from build123d import *

# Parameters (mm, degrees)
SKETCH_1_R             = 60
SM_BASE_FLANGE_1_DEPTH = 2
CUT_EXTRUDE_1_REACH    = 86.876
SKETCH_6_R             = 1.5


# Sheet-metal steps are written as plain solids
with BuildPart() as part:
    # Sketch 1 → 基体-法兰1 (new body)
    with BuildSketch(Plane(origin=(0, 0, 0), x_dir=(1, 0, 0), z_dir=(0, 1, 0))):
        with Locations(Location((0, 0, 0), (0, 0, 270))):
            Circle(SKETCH_1_R)
        with BuildLine():
            Line((-5.662691153, -45.650125179), (-5.41648719, -43.665337128))
            ThreePointArc((-5.41648719, -43.665337128), (-0.000329002, 43.999999999), (5.41714019, -43.665256122))
            Line((5.41714019, -43.665256122), (5.663373835, -45.650040491))
            ThreePointArc((5.663373835, -45.650040491), (0.000343957, -45.999999999), (-5.662691153, -45.650125179))
        make_face(mode=Mode.SUBTRACT)
    extrude(amount=-SM_BASE_FLANGE_1_DEPTH)

    # 草图6 → 切除-拉伸1 (cut, up to next)
    with BuildSketch(Plane(origin=(0, 0, 0), x_dir=(1, 0, 0), z_dir=(0, 1, 0)), mode=Mode.PRIVATE) as cut_extrude_1_sk1:
        with Locations(Location((36.769552622, 36.769552622, 0), (0, 0, 270))):
            Circle(SKETCH_6_R)
    cut_extrude_1_tool1 = extrude(cut_extrude_1_sk1.sketch, amount=-CUT_EXTRUDE_1_REACH, mode=Mode.PRIVATE) & part.part
    # 草图6 → 切除-拉伸1 (cut, up to next)
    with BuildSketch(Plane(origin=(0, 0, 0), x_dir=(1, 0, 0), z_dir=(0, 1, 0)), mode=Mode.PRIVATE) as cut_extrude_1_sk2:
        with Locations(Location((-36.769552622, 36.769552622, 0), (0, 0, 270))):
            Circle(SKETCH_6_R)
    cut_extrude_1_tool2 = extrude(cut_extrude_1_sk2.sketch, amount=-CUT_EXTRUDE_1_REACH, mode=Mode.PRIVATE) & part.part
    # 草图6 → 切除-拉伸1 (cut, up to next)
    with BuildSketch(Plane(origin=(0, 0, 0), x_dir=(1, 0, 0), z_dir=(0, 1, 0)), mode=Mode.PRIVATE) as cut_extrude_1_sk3:
        with Locations(Location((36.769552622, -36.769552622, 0), (0, 0, 270))):
            Circle(SKETCH_6_R)
    cut_extrude_1_tool3 = extrude(cut_extrude_1_sk3.sketch, amount=-CUT_EXTRUDE_1_REACH, mode=Mode.PRIVATE) & part.part
    # 草图6 → 切除-拉伸1 (cut, up to next)
    with BuildSketch(Plane(origin=(0, 0, 0), x_dir=(1, 0, 0), z_dir=(0, 1, 0)), mode=Mode.PRIVATE) as cut_extrude_1_sk4:
        with Locations(Location((-36.769552622, -36.769552622, 0), (0, 0, 270))):
            Circle(SKETCH_6_R)
    cut_extrude_1_tool4 = extrude(cut_extrude_1_sk4.sketch, amount=-CUT_EXTRUDE_1_REACH, mode=Mode.PRIVATE) & part.part
    add(cut_extrude_1_tool1.solids().sort_by_distance((36.769553, 0, -36.769553))[0], mode=Mode.SUBTRACT)
    add(cut_extrude_1_tool2.solids().sort_by_distance((-36.769553, 0, -36.769553))[0], mode=Mode.SUBTRACT)
    add(cut_extrude_1_tool3.solids().sort_by_distance((36.769553, 0, 36.769553))[0], mode=Mode.SUBTRACT)
    add(cut_extrude_1_tool4.solids().sort_by_distance((-36.769553, 0, 36.769553))[0], mode=Mode.SUBTRACT)


solid = part.part
Model file for the job. Use its own axes, mm. Round coordinates to 2 decimals unless told otherwise and drop trailing zeros. Loops run counter-clockwise (first coordinate to the right, second up) from the corner with the lowest first, then second, coordinate; pieces in that order, holes last.
1. Band-saw the part on A-A, the plane x = 0. List the corners of the cut face in (y, z), and give its area (3 significant figures).
Check values:
outline: (-2, -60) - (0, -60) - (0, -44) - (-2, -44) - close; (-2, 46) - (0, 46) - (0, 60) - (-2, 60) - close
area: 60.0 mm2
2. Band-saw the part on C-C, the plane y = -1.5. List the corners of the cut face in (x, z).
Check values:
outline: circle Ø120 at (0, 0); hole circle Ø3 at (-36.77, -36.77); hole circle Ø3 at (-36.77, 36.77); hole (-5.66, 45.65) - (-5.42, 43.67) arc R44 ccw (long way) to (5.42, 43.67) - (5.66, 45.65) arc R46 ccw to start; hole circle Ø3 at (36.77, -36.77); hole circle Ø3 at (36.77, 36.77)
3. Wall check: probe 1 along X at (y, z) = (-1, 0); probe 2 along Z at (x, y) = (-37, -0.55); probe 3 along X at (y, z) = (-0.7, 14.5). Give the ranges that are in metal, low to high.
Check values:
probe 1: x = -60 to -44, 44 to 60
probe 2: z = -47.23 to -38.25, -35.29 to -23.81, 23.81 to 35.29, 38.25 to 47.23
probe 3: x = -58.22 to -41.54, 41.54 to 58.22
4. Band-saw the part on B-B, the plane z = 0. List the corners of the cut face in (x, y).
Check values:
outline: (-60, -2) - (-44, -2) - (-44, 0) - (-60, 0) - close; (44, -2) - (60, -2) - (60, 0) - (44, 0) - close
5. Mould opens along Z. For faces 1 (the cylindrical face through (2.64, -0.99, -59.94)), 2 (the flat face through (31.4, 0, -31.4)), 3 (the cylindrical face through (-1.86, -0.99, -43.96)) say: +Z half, -Z half, draft (parallel to the pull), parting line (faces both ways), or undercut.
Check values:
face 1: parting line
face 2: draft
face 3: undercut
6. Drop flat-ended pins along their axis: P1, Ø2.5, axis at x = 36.77, z = -36.77, coming from the -Y side; P2, Ø5, axis at x = -36.77, z = 36.77, coming from the -Y side; P3, Ø1, axis at y = -1, z = -29.5, coming from the +X side; P4, Ø1, axis at x = -21.5, y = -1.5, coming from the -Z side (3 decimals). Give the stop position or say it passes through.
Check values:
P1: passes through
P2: stops at y = -2
P3: stops at x = 52.53
P4: stops at z = -56.205
7. Band-saw the part on D-D, the plane z = -49. List the corners of the cut face in (x, y), and give its area (3 significant figures).
Check values:
outline: (-34.63, -2) - (34.63, -2) - (34.63, 0) - (-34.63, 0) - close
area: 139 mm2
